Work out the finished part from the listing and answer in its coordinate system (mm). A direction names the side the tool comes from. Coordinates: 2 decimals unless noted, no trailing zeros. Loops run counter-clockwise (first coordinate to the right, second up) from the corner with the lowest first, then second, coordinate; pieces in that order, holes last.
```python
from build123d import *

# Parameters (mm, degrees)
SKETCH_1_R                      = 12.55
EXTRUDE_1_DEPTH                 = 6
SKETCH_2_R                      = 3.2
CUT_EXTRUDE_1_DEPTH             = 6
CUT_EXTRUDE_2_REACH             = 20.735
SKETCH_3_R                      = 1
CUT_EXTRUDE_2_DIRECTION_2_REACH = 20.735
EXTRUDE_2_DEPTH                 = 2.5
EXTRUDE_2_DEPTH_BACK            = 1
SKETCH_4_R                      = 15
SKETCH_5_R                      = 13.5
CUT_EXTRUDE_3_DEPTH             = 2.5
FILLET_2_R                      = 2
SKETCH_7_W                      = 2.5
SKETCH_7_H                      = 10
CUT_EXTRUDE_4_DEPTH             = 21


with BuildPart() as part:
    # 草图1 → 凸台-拉伸1 (new body)
    with BuildSketch(Plane(origin=(0, 0, 0), x_dir=(0, 0, -1), z_dir=(1, 0, 0))):
        Circle(SKETCH_1_R)
    extrude(amount=EXTRUDE_1_DEPTH)

    # 草图2 → 切除-拉伸1 (cut)
    with BuildSketch(Plane.ZY):
        Circle(SKETCH_2_R)
    extrude(amount=-CUT_EXTRUDE_1_DEPTH, mode=Mode.SUBTRACT)

    # 草图3 → 切除-拉伸2 (cut, up to next)
    with BuildSketch(Plane(origin=(0, 0, 0), x_dir=(1, 0, 0), z_dir=(0, 1, 0)), mode=Mode.PRIVATE) as cut_extrude_2_sk1:
        with Locations(Location((3, 0, 0), (0, 0, 270))):
            Circle(SKETCH_3_R)
    cut_extrude_2_tool1 = extrude(cut_extrude_2_sk1.sketch, amount=-CUT_EXTRUDE_2_REACH, mode=Mode.PRIVATE) & part.part
    add(cut_extrude_2_tool1.solids().sort_by_distance((3, 0, 0))[0], mode=Mode.SUBTRACT)

    # 草图3 → 切除-拉伸2 direction 2 (cut, up to next)
    with BuildSketch(Plane(origin=(0, 0, 0), x_dir=(1, 0, 0), z_dir=(0, 1, 0)), mode=Mode.PRIVATE) as cut_extrude_2_direction_2_sk1:
        with Locations(Location((3, 0, 0), (0, 0, 270))):
            Circle(SKETCH_3_R)
    cut_extrude_2_direction_2_tool1 = extrude(cut_extrude_2_direction_2_sk1.sketch, amount=CUT_EXTRUDE_2_DIRECTION_2_REACH, mode=Mode.PRIVATE) & part.part
    add(cut_extrude_2_direction_2_tool1.solids().sort_by_distance((3, 0, 0))[0], mode=Mode.SUBTRACT)

    # 草图4 → 凸台-拉伸2 (add, two sides: drawn at the far end of the back side and taken through both)
    with BuildSketch(Plane(origin=(6, 0, 0), x_dir=(0, 0, -1), z_dir=(1, 0, 0)).offset(-EXTRUDE_2_DEPTH_BACK)):
        Circle(SKETCH_4_R)
    extrude(amount=EXTRUDE_2_DEPTH + EXTRUDE_2_DEPTH_BACK)

    # 草图5 → 切除-拉伸3 (cut)
    with BuildSketch(Plane(origin=(8.5, 0, 0), x_dir=(0, 0, -1), z_dir=(1, 0, 0))):
        Circle(SKETCH_5_R)
    extrude(amount=-CUT_EXTRUDE_3_DEPTH, mode=Mode.SUBTRACT)

    # 圆角2
    # the kernel refuses this fillet: 2 mm, written as the material it adds along each edge
    with BuildSketch(Plane(origin=(5, 0, 0), x_dir=(0, 0, -1), z_dir=(0, 1, 0))) as fillet_2_piece_1_section:
        with BuildLine():
            CenterArc((12.55 + FILLET_2_R, FILLET_2_R), FILLET_2_R, 180, 90)
            Line((12.55 + FILLET_2_R, 0), (12.55, 0))
            Line((12.55, 0), (12.55, FILLET_2_R))
        make_face()
    fillet_2_piece_1 = revolve(axis=Axis((5, 0, 0), (-1, 0, 0)), mode=Mode.PRIVATE)
    fillet_2_piece_1 = fillet_2_piece_1 - Plane(origin=(3, 0, 0), x_dir=(0, 0, 1), z_dir=(0, -1, 0)) * Cylinder(1, 59, mode=Mode.PRIVATE)
    add(fillet_2_piece_1)

    # 草图7 → 切除-拉伸4 (cut)
    with BuildSketch(Plane(origin=(0, 0, 0), x_dir=(1, 0, 0), z_dir=(0, 1, 0))):
        with Locations((7.25, 0)):
            Rectangle(SKETCH_7_W, SKETCH_7_H)
    extrude(amount=-CUT_EXTRUDE_4_DEPTH, mode=Mode.SUBTRACT)


solid = part.part
```
1. For faces 4 (the flat face through (0, -3, -3)), 5 (the cylindrical face through (6.73, 12.65, -8.06)), 6 (the flat face through (5, 0, 0)), 7 (the cylindrical face through (7.27, 13.49, -0.52)), 8 (the flat face through (7, -13, -5)), determine the directions among +Z, -Z, +X, -X, +Y, -Y from which every point of the face is accessible in a straight line to the end or side of a thin tool.
2. A cutting plane is placed at A-A, the plane z = 0. Give the vertices of the cut face in (x, y), then the cut area to 3 significant figures.
3. Each of these flat-tipped pins is pushed along its axis until it touches: P1, Ø5, axis at y = 0, z = -1, coming from the -X side; P2, Ø1, axis at x = 4, z = -5.5, coming from the +Y side; P3, Ø2.5, axis at x = 3, z = 0, coming from the -Y side; P4, Ø0.5, axis at x = 7.5, y = -13, coming from the -Z side. Where does it stop, or does it pass through?
4. A cutting plane is placed at C-C, the plane x = 1.5. Give the vertices of the cut face in (y, z).
5. Determine the mould class of faces 1 (the cylindrical face through (2.465, 0.961, 3.052)), 2 (the cylindrical face through (1.48, -4.81, -11.59)), 3 (the flat face through (8.5, 13.4, 3.4)) for opening direction Y: released by +Y, released by -Y, zero draft, split by the parting line, or undercut.
6. A cutting plane is placed at D-D, the plane x = 7. Give the vertices of the cut face in (y, z).
7. Straight lines are drawn through the part: probe 1 along X at (y, z) = (6, 0); probe 2 along X at (y, z) = (-4, 9.5); probe 3 along X at (y, z) = (1, -0.5). For each, find the intervals that lie inside material, in ascending order.
8. A cutting plane is placed at B-B, the plane y = 0. Give the vertices of the cut face in (x, z).
Answers below:
1. face 4: +Z, -Z, -X, +Y, -Y
1. face 5: +X, -X
1. face 6: -X
1. face 7: +X
1. face 8: +X, -Y
2. outline: (0, -12.55) - (2, -12.55) - (2, -3.2) - (0, -3.2) - close; (0, 3.2) - (2, 3.2) - (2, 12.55) - (0, 12.55) - close; (4, -12.82) arc R2 cw to (5, -14.55) - (5, -15) - (6, -15) - (6, 13.5) - (8.5, 13.5) - (8.5, 15) - (5, 15) - (5, 14.55) arc R2 cw to (4, 12.82) - (4, 3.2) - (5, 3.2) - (5, -3.2) - (4, -3.2) - close
2. area: 91.4 mm2
3. P1: stops at x = 0
3. P2: stops at y = 12.07
3. P3: stops at y = -12.99
3. P4: stops at z = -7.9
4. outline: circle Ø25.1 at (0, 0); hole circle Ø6.4 at (0, 0)
5. face 1: undercut
5. face 2: split by the parting line
5. face 3: zero draft
6. outline: (-14.14, -5) arc R15 ccw (long way) to (-14.14, 5) - (-12.54, 5) arc R13.5 cw (long way) to (-12.54, -5) - close
7. probe 1: x = 0 to 2, 4 to 6
7. probe 2: x = 0 to 6
7. probe 3: x = 5 to 6
8. outline: (0, -12.55) - (3, -12.55) arc R2 cw to (5, -14.55) - (5, -15) - (8.5, -15) - (8.5, -13.5) - (6, -13.5) - (6, 13.5) - (8.5, 13.5) - (8.5, 15) - (5, 15) - (5, 14.55) arc R2 cw to (3, 12.55) - (0, 12.55) - (0, 3.2) - (5, 3.2) - (5, -3.2) - (0, -3.2) - close
